```python
from build123d import *

# Parameters (mm, degrees)
BOSS_EXTRUDE1_DEPTH = 10
BOSS_EXTRUDE2_DEPTH = 2
CUT_EXTRUDE1_START  = -6.4
CUT_EXTRUDE1_DEPTH  = 1.4


with BuildPart() as part:
    # Sketch1 → Boss-Extrude1 (new body)
    with BuildSketch(Plane(origin=(0, 0, 0), x_dir=(1, 0, 0), z_dir=(0, 1, 0))):
        with BuildLine():
            Line((-42.5, -117.5), (42.5, -117.5))
            ThreePointArc((42.5, -117.5), (46.035533906, -116.035533906), (47.5, -112.5))
            Line((47.5, -112.5), (47.5, 112.5))
            ThreePointArc((47.5, 112.5), (46.035533906, 116.035533906), (42.5, 117.5))
            Line((42.5, 117.5), (-42.5, 117.5))
            ThreePointArc((-42.5, 117.5), (-46.035533906, 116.035533906), (-47.5, 112.5))
            Line((-47.5, 112.5), (-47.5, -112.5))
            ThreePointArc((-47.5, -112.5), (-46.035533906, -116.035533906), (-42.5, -117.5))
        make_face()
    extrude(amount=BOSS_EXTRUDE1_DEPTH)

    # Sketch2 → Boss-Extrude2 (add)
    with BuildSketch(Plane.XZ):
        with BuildLine():
            Line((-48.4, 112.5), (-48.4, -112.5))
            ThreePointArc((-48.4, -112.5), (-46.671930009, -116.671930009), (-42.5, -118.4))
            Line((-42.5, -118.4), (42.5, -118.4))
            ThreePointArc((42.5, -118.4), (46.671930009, -116.671930009), (48.4, -112.5))
            Line((48.4, -112.5), (48.4, 112.5))
            ThreePointArc((48.4, 112.5), (46.671930009, 116.671930009), (42.5, 118.4))
            Line((42.5, 118.4), (-42.5, 118.4))
            ThreePointArc((-42.5, 118.4), (-46.671930009, 116.671930009), (-48.4, 112.5))
        make_face()
    extrude(amount=BOSS_EXTRUDE2_DEPTH)

    # Sketch3 → Cut-Extrude1 (cut)
    with BuildSketch(Plane(origin=(0, 10, 0), x_dir=(1, 0, 0), z_dir=(0, 1, 0)).offset(CUT_EXTRUDE1_START)):
        with BuildLine():
            Line((-47.5, 112.5), (-47.5, -112.5))
            ThreePointArc((-47.5, -112.5), (-46.035533906, -116.035533906), (-42.5, -117.5))
            Line((-42.5, -117.5), (42.5, -117.5))
            ThreePointArc((42.5, -117.5), (46.035533906, -116.035533906), (47.5, -112.5))
            Line((47.5, -112.5), (47.5, 112.5))
            ThreePointArc((47.5, 112.5), (46.035533906, 116.035533906), (42.5, 117.5))
            Line((42.5, 117.5), (-42.5, 117.5))
            ThreePointArc((-42.5, 117.5), (-46.035533906, 116.035533906), (-47.5, 112.5))
        make_face()
        with BuildLine():
            ThreePointArc((-42.5, 116.8), (-45.540559159, 115.540559159), (-46.8, 112.5))
            Line((-46.8, 112.5), (-46.8, -112.5))
            ThreePointArc((-46.8, -112.5), (-45.540559159, -115.540559159), (-42.5, -116.8))
            Line((-42.5, -116.8), (42.5, -116.8))
            ThreePointArc((42.5, -116.8), (45.540559159, -115.540559159), (46.8, -112.5))
            Line((46.8, -112.5), (46.8, 112.5))
            ThreePointArc((46.8, 112.5), (45.540559159, 115.540559159), (42.5, 116.8))
            Line((42.5, 116.8), (-42.5, 116.8))
        make_face(mode=Mode.SUBTRACT)
    extrude(amount=CUT_EXTRUDE1_DEPTH, mode=Mode.SUBTRACT)


solid = part.part
```
Could you check a few things on this model? Use its own coordinates, in mm. A direction names the side the tool comes from. Coordinates: 2 decimals unless noted, no trailing zeros. Loops run counter-clockwise (first coordinate to the right, second up) from the corner with the lowest first, then second, coordinate; pieces in that order, holes last. Notation, with made-up numbers: M -34,-37 L 1,-37 A29 cw 1,-8 Z; hole C 50.25,14 d7. An arc over 180 degrees is marked long. Put each result on its own line as item: value. Start each with the question number.
(1) For faces 1 (the face through (46.07, 1.77, -116)), 2 (the face through (46, 7.46, 116.07)), 3 (the face through (47.5, 7, 2)), 4 (the face through (-47.5, 7, -2)), which set-ups out of +Z, -Z, +X, -X, +Y, -Y let a thin tool reach every point of the face, with its end or its side?
(2) Suppose I cut it at A-A on z = -98. Please give me the cut outline in (x, y), then the cut area to 3 significant figures.
(3) I need wall thicknesses on line 1 (Z direction, x = -19.5, y = 7); line 2 (X direction, y = 3.5, z = -32.5); line 3 (X direction, y = 4.5, z = 85.5). Which ranges of each line are inside material? Lowest first, please. Write a range as from..to.
(4) Thinking about a two-plate mould opening in Y: for faces 5 (the face through (-1, 10, -2)), 6 (the face through (-1, -2, 2)), 7 (the face through (-45.51, 4.29, -115.57)), which applies, pulls with the +Y half, pulls with the -Y half, needs draft (parallel to the pull), parting line crosses it, or undercut?
(5) Will these pins go through, and if not, where does the flat tip stop? P1, Ø0.7, axis at y = 4.5, z = -51.5, coming from the -X side; P2, Ø4, axis at y = 2.5, z = -3, coming from the +X side; P3, Ø4, axis at x = -3, y = 8.5, coming from the -Z side; P4, Ø4, axis at y = 0.5, z = -43.5, coming from the +X side.
Solutions:
1. face 1: -Z, +X, +Y
1. face 2: +Z, +X, +Y
1. face 3: +Z, -Z, +X, +Y
1. face 4: +Z, -Z, -X, +Y
2. outline: M -48.4,-2 L 48.4,-2 L 48.4,0 L 47.5,0 L 47.5,3.6 L 46.8,3.6 L 46.8,5 L 47.5,5 L 47.5,10 L -47.5,10 L -47.5,5 L -46.8,5 L -46.8,3.6 L -47.5,3.6 L -47.5,0 L -48.4,0 Z
2. area: 1,140 mm2
3. line 1: z = -117.5..117.5
3. line 2: x = -47.5..47.5
3. line 3: x = -46.8..46.8
4. face 5: pulls with the +Y half
4. face 6: pulls with the -Y half
4. face 7: undercut
5. P1: stops at x = -46.8
5. P2: stops at x = 47.5
5. P3: stops at z = -117.5
5. P4: stops at x = 48.4
